Could you check a few things on this drawing? It's one solid part, dimensions in mm from its lowest x, y, z. Give positions to 0.01 mm unless a question says otherwise; leave off trailing zeros. Loops run counter-clockwise (first coordinate to the right, second up) from the corner with the lowest first, then second, coordinate; pieces in that order, holes last. Notation, with made-up numbers: (53.5, 11.25) - (87.5, 11.25) arc R22 cw to (87.5, 42.25) - close; hole circle Ø10 at (59.5, 54.5). An arc over 180 degrees is marked (long way). Return JSON: item names as keys, results as strings. Group by question number.
(1) If we section it at A-A (y = 210): Please give me the cut outline in (x, z), then the cut area to 3 significant figures.
(2) If we section it at B-B (y = 110): Please give me the cut outline in (x, z), then the cut area to 3 significant figures.
(3) If we section it at C-C (x = 150): Please give me the cut outline in (y, z), then the cut area to 3 significant figures.
(4) I need wall thicknesses on probe 1 along Y at (x, z) = (70, 5.5); probe 2 along X at (y, z) = (180, 3); probe 3 along X at (y, z) = (210.5, 3). Which ranges of each line are inside material? Lowest first, please. Write a range as [from, to].
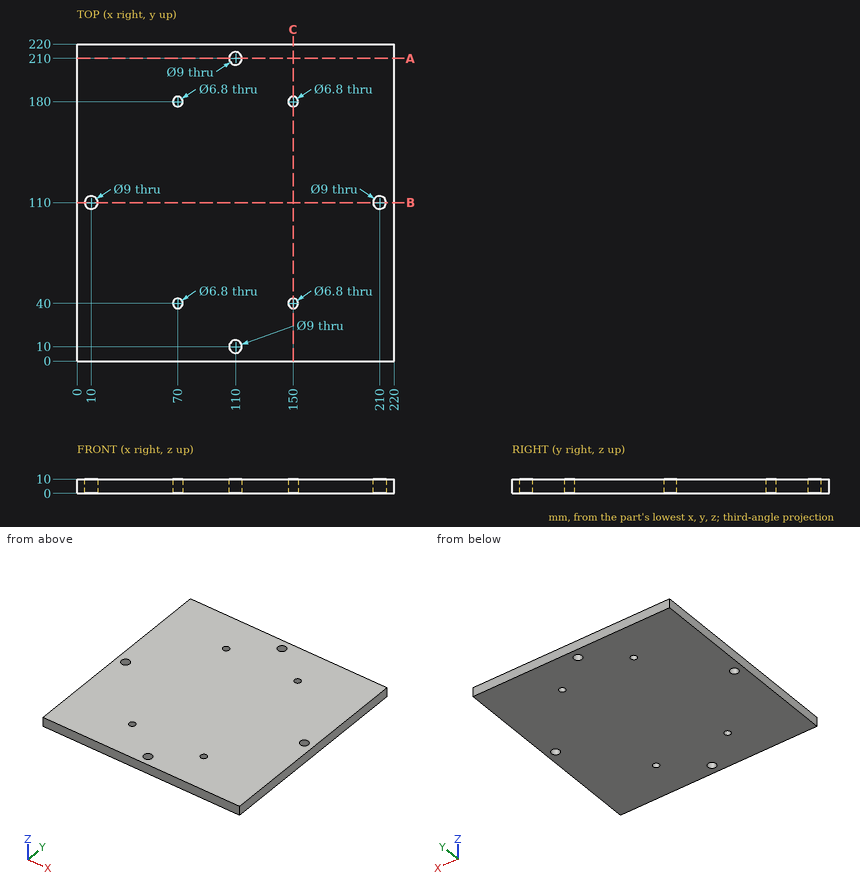
Values:
{
 "1": {"outline": "(0, 0) - (105.5, 0) - (105.5, 10) - (0, 10) - close; (114.5, 0) - (220, 0) - (220, 10) - (114.5, 10) - close", "area": "2,110 mm2"},
 "2": {"outline": "(0, 0) - (5.5, 0) - (5.5, 10) - (0, 10) - close; (14.5, 0) - (205.5, 0) - (205.5, 10) - (14.5, 10) - close; (214.5, 0) - (220, 0) - (220, 10) - (214.5, 10) - close", "area": "2,020 mm2"},
 "3": {"outline": "(0, 0) - (36.6, 0) - (36.6, 10) - (0, 10) - close; (43.4, 0) - (176.6, 0) - (176.6, 10) - (43.4, 10) - close; (183.4, 0) - (220, 0) - (220, 10) - (183.4, 10) - close", "area": "2,060 mm2"},
 "4": {"probe 1": "[0, 36.6], [43.4, 176.6], [183.4, 220]", "probe 2": "[0, 66.6], [73.4, 146.6], [153.4, 220]", "probe 3": "[0, 105.53], [114.47, 220]"}
}
